Design review of the part shown in the three views and the two pictorial views. Dimensions are in mm from the part's minimum x, y and z. Give positions to 0.01 mm unless a question says otherwise; leave off trailing zeros. Write each loop counter-clockwise with the first axis right and the second up, starting at its lowest first coordinate (ties: lowest second). Pieces come first, ordered by that corner, then holes. Notation, with made-up numbers: M 84.5,28 L 127.5,28 A16 cw 127.5,43 Z; hole C 78.25,-32 d9. An arc over 180 degrees is marked long. Use one line per item in the form item = value. Start each with the question number.
Q1. Mouldability with a two-part tool opening along X and no side actions: class the marked faces 1, 2 and 3 as released by +X, released by -X, zero draft, split by the parting line, or undercut.
Q2. Clearance check with flat-ended pins moving along their axes: pin 1 Ø1.5 at (x, z) = (58.5, 18.5) entering from +Y; pin 2 Ø1 at (x, y) = (18.5, 5.5) entering from -Z; pin 3 Ø8.5 at (x, y) = (10.5, 12.5) entering from -Z. State where each tip first meets the part, or that it passes through.
Q3. Consider section B-B on x = 41.05. Write out the cut boundary in (y, z).
Q4. For probe 1 along X at (y, z) = (5, 78.75); probe 2 along X at (y, z) = (11.75, 15); probe 3 along Z at (x, y) = (41.05, 3.25), list the stretches that pass through material, from the lowest coordinate up. Write a range as [from, to].
Q5. Consider section C-C on z = 48. Write out the cut boundary in (x, y).
Q6. Consider section D-D on x = 10. Write out the cut boundary in (y, z), and give its area (3 significant figures).
Q7. Consider section A-A on z = 78.75. Write out the cut boundary in (x, y).
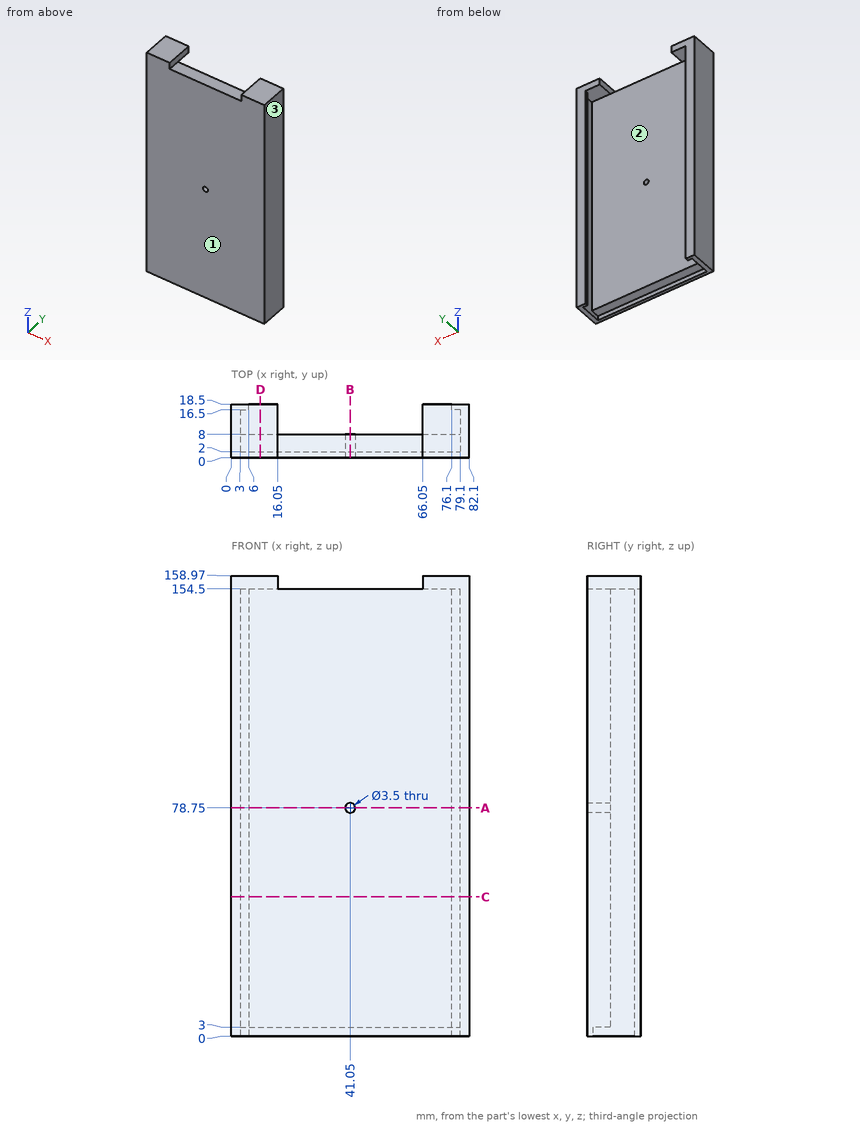
Working result:
q1.face_1 = zero draft
q1.face_2 = undercut
q1.face_3 = released by +X
q2.pin_1 = 8
q2.pin_2 = 3
q2.pin_3 = 154.5
q3.outline = M 0,0 L 2,0 L 2,3 L 8,3 L 8,77 L 0,77 Z; M 0,80.5 L 8,80.5 L 8,154.5 L 0,154.5 Z
q4.probe_1 = [0, 39.3], [42.8, 82.1]
q4.probe_2 = [0, 3], [79.1, 82.1]
q4.probe_3 = [3, 77], [80.5, 154.5]
q5.outline = M 0,0 L 82.1,0 L 82.1,18.5 L 76.1,18.5 L 76.1,16.5 L 79.1,16.5 L 79.1,8 L 3,8 L 3,16.5 L 6,16.5 L 6,18.5 L 0,18.5 Z
q6.outline = M 0,0 L 2,0 L 2,3 L 8,3 L 8,154.5 L 18.5,154.5 L 18.5,158.97 L 0,158.97 Z
q6.area = 1,300 mm²
q7.outline = M 0,0 L 39.3,0 L 39.3,8 L 3,8 L 3,16.5 L 6,16.5 L 6,18.5 L 0,18.5 Z; M 42.8,0 L 82.1,0 L 82.1,18.5 L 76.1,18.5 L 76.1,16.5 L 79.1,16.5 L 79.1,8 L 42.8,8 Z
